from build123d import *

# Parameters (mm, degrees)
CROQUIS1_R                 = 13
CROQUIS1_R_2               = 4.6
SALIENTE_EXTRUIR1_DEPTH    = 40
CROQUIS1_2_R               = 13
CROQUIS1_2_R_2             = 4.6
SALIENTE_EXTRUIR2_DEPTH    = 16
CROQUIS2_R                 = 6.5
SALIENTE_EXTRUIR3_DEPTH    = 22
REDONDEO1_R                = 0.5
REDONDEO2_R                = 0.5
CROQUIS3_R                 = 2.75
CORTAR_EXTRUIR1_DEPTH      = 45.022721406
CORTAR_EXTRUIR1_DEPTH_BACK = 45.022721406


with BuildPart() as part:
    # Croquis1 → Saliente-Extruir1 (new body)
    with BuildSketch(Plane.XY):
        Circle(CROQUIS1_R)
        Circle(CROQUIS1_R_2, mode=Mode.SUBTRACT)
    extrude(amount=SALIENTE_EXTRUIR1_DEPTH)

    # Croquis1_2 → Saliente-Extruir2 (add)
    with BuildSketch(Plane.XY):
        Circle(CROQUIS1_2_R)
        Circle(CROQUIS1_2_R_2, mode=Mode.SUBTRACT)
        Circle(CROQUIS1_2_R_2)
    extrude(amount=-SALIENTE_EXTRUIR2_DEPTH)

    # Croquis2 → Saliente-Extruir3 (add)
    with BuildSketch(Plane(origin=(0, 0, -16), x_dir=(-1, 0, 0), z_dir=(0, 0, -1))):
        Circle(CROQUIS2_R)
    extrude(amount=SALIENTE_EXTRUIR3_DEPTH)

    # Redondeo1
    redondeo1_edges = [part.edges().sort_by_distance(p)[0] for p in [
        (6.5, 0, -16),
    ]]
    fillet(redondeo1_edges, radius=REDONDEO1_R)

    # Redondeo2
    redondeo2_edges = [part.edges().sort_by_distance(p)[0] for p in [
        (-4.6, 0, 0),
    ]]
    fillet(redondeo2_edges, radius=REDONDEO2_R)

    # Croquis3 → Cortar-Extruir1 (cut, two sides)
    with BuildSketch(Plane(origin=(0, 0, 0), x_dir=(1, 0, 0), z_dir=(0, 1, 0))) as cortar_extruir1_sk:
        with Locations(Location((0, 9.25, 0), (0, 0, 270))):
            Circle(CROQUIS3_R)
    extrude(amount=CORTAR_EXTRUIR1_DEPTH, mode=Mode.SUBTRACT)
    extrude(cortar_extruir1_sk.sketch, amount=-CORTAR_EXTRUIR1_DEPTH_BACK, mode=Mode.SUBTRACT)


solid = part.part
For this review, take the finished solid that the model builds, in its own axes (mm). A direction names the side the tool comes from. Give positions to 0.01 mm unless a question says otherwise; leave off trailing zeros. Loops run counter-clockwise (first coordinate to the right, second up) from the corner with the lowest first, then second, coordinate; pieces in that order, holes last. Notation, with made-up numbers: M -39,5.25 L 12,5.25 A15 cw 12,31.25 Z; hole C 87,25.5 d4. An arc over 180 degrees is marked long. Put each result on its own line as item: value. Start each with the question number.
(1) The part is to be moulded in two halves that separate along Z. For faces 1 (the cylindrical face through (5.158, -3.955, -27.1)), 2 (the cylindrical face through (-1.05, 0.18, -6.71)), 3 (the flat face through (0, 0, -38)), 4 (the flat face through (0, 0, 0)), say which applies: +Z half, -Z half, draft (parallel to the pull), parting line (faces both ways), or undercut.
(2) Add section A-A, the plane x = 0. Write out the cut boundary in (y, z), then the cut area to 3 significant figures.
(3) Add section D-D, the plane z = 15.5. Write out the cut boundary in (x, y).
(4) Add section B-B, the plane y = 0. Write out the cut boundary in (x, z), then the cut area to 3 significant figures.
(5) Machinability: for faces 5 (the flat face through (6, -6, -16)), 6 (the flat face through (6, 0, 40)), 7 (the cylindrical face through (-3.65, -2.8, 19.97)), which of the approach directions +Z, -Z, +X, -X, +Y, -Y give a long, thin tool a straight path to every point of the face, cutting with its end or side? Answer none if there is none.
(6) Wall thickness on L1, parallel to Z at x = 0, y = 6.25; L2, parallel to Z at x = 0, y = 7.25; L3, parallel to Y at x = 0.25, z = 27.5: over which ranges is each line inside the solid? List them lowest first.
(7) Add section C-C, the plane z = -13.5. Write out the cut boundary in (x, y).
(8) For pin 1 (8 mm diameter, centred on x = 7, z = 24, fed in from -Y); pin 2 (3 mm diameter, centred on y = 7.5, z = 12, fed in from +X); pin 3 (3 mm diameter, centred on x = -5, z = -12.5, fed in from -Y), all flat-tipped, find the tip position at first contact; note any pin that passes through.
Result:
1. face 1: draft
1. face 2: undercut
1. face 3: -Z half
1. face 4: +Z half
2. outline: M -13,-16 L -7,-16 A0.5 cw -6.5,-16.5 L -6.5,-38 L 6.5,-38 L 6.5,-16.5 A0.5 cw 7,-16 L 13,-16 L 13,-12 L -13,-12 Z; M -13,-6.5 L 13,-6.5 L 13,40 L 4.6,40 L 4.6,0.5 A0.5 cw 4.1,0 L -4.1,0 A0.5 cw -4.6,0.5 L -4.6,40 L -13,40 Z
2. area: 1,230 mm^2
3. outline: C 0,0 d26; hole C 0,0 d9.2
4. outline: M -13,-16 L -7,-16 A0.5 cw -6.5,-16.5 L -6.5,-38 L 6.5,-38 L 6.5,-16.5 A0.5 cw 7,-16 L 13,-16 L 13,40 L 4.6,40 L 4.6,0.5 A0.5 cw 4.1,0 L -4.1,0 A0.5 cw -4.6,0.5 L -4.6,40 L -13,40 Z; hole C 0,-9.25 d5.5
4. area: 1,350 mm^2
5. face 5: -Z
5. face 6: +Z, +X, -X, +Y, -Y
5. face 7: +Z
6. L1: z = -38 to -12, -6.5 to 40
6. L2: z = -16 to -12, -6.5 to 40
6. L3: y = -13 to -4.59, 4.59 to 13
7. outline: C 0,0 d26
8. pin 1: stops at y = -12.65
8. pin 2: stops at x = 11.53
8. pin 3: stops at y = -12.52
